```python
from build123d import *

# Parameters (mm, degrees)
F0_W          = 7
F0_H          = 100
F1_DEPTH      = 75
F1_DEPTH_BACK = 75
F2_W          = 7
F2_H          = 125
F3_DEPTH      = 5
F5_R          = 25
F6_R          = 3


with BuildPart() as f1:
    # F0 (on Right) → F1 (new body, two sides)
    with BuildSketch(Plane.YZ) as f1_sk:
        Rectangle(F0_W, F0_H)
    extrude(amount=F1_DEPTH)
    extrude(f1_sk.sketch, amount=-F1_DEPTH_BACK)

    # F2 (on face) → F3 (join)
    with BuildSketch(Plane.YZ.offset(75)):
        with Locations((0, -12.5)):
            Rectangle(F2_W, F2_H)
    extrude(amount=F3_DEPTH)

    # F4: F1 across plane


with BuildPart() as f1_1:
    add(f1.part)
    add(f1.part.mirror(Plane.YZ))

    # F5
    f5_edges = [f1_1.edges().sort_by_distance(p)[0] for p in [
        (-80, 0, 50),
        (80, 0, 50),
    ]]
    fillet(f5_edges, radius=F5_R)

    # F6
    f6_edges = [f1_1.edges().sort_by_distance(p)[0] for p in [
        (-77.5, -3.5, -75),
        (77.5, -3.5, -75),
        (-77.5, 3.5, -75),
        (77.5, 3.5, -75),
    ]]
    fillet(f6_edges, radius=F6_R)


solid = f1_1.part
```
Geometry check sheet. Reference: the model listing, model coordinates, mm. A direction names the side the tool comes from. Round coordinates to 2 decimals unless told otherwise and drop trailing zeros. Loops run counter-clockwise (first coordinate to the right, second up) from the corner with the lowest first, then second, coordinate; pieces in that order, holes last. Notation, with made-up numbers: (61, 54) -> (81, 54) arc R19 cw to (81, 79) -> close; hole circle Ø6 at (61.5, -17). An arc over 180 degrees is marked (long way). Use a Markdown table: item, result.
(1) Sectioned sample at D-D (z = 42.5). Enter the section's corners in (x, y), then the cut area to 3 significant figures.
Calculated:
| item | result |
|---|---|
| outline | (-72.85, -3.5) -> (72.85, -3.5) -> (72.85, 3.5) -> (-72.85, 3.5) -> close |
| area | 1,020 mm² |
(2) Mould release check, pull along X, two halves, no side actions. Record for faces 3 (the flat face through (1, 3.5, 2)), 4 (the flat face through (80, 0, -24)), 5 (the flat face through (-75, 0, -62)), 6 (the flat face through (75, 0, -62)): released by +X, released by -X, zero draft, split by the parting line, or undercut.
Calculated:
| item | result |
|---|---|
| face 3 | zero draft |
| face 4 | released by +X |
| face 5 | undercut |
| face 6 | undercut |
(3) Set-up check for faces 1 (the cylindrical face through (72.871, 0.049, 42.482)), 2 (the flat face through (1, 0, -50)): record each of +Z, -Z, +X, -X, +Y, -Y from which the full face is reachable in a straight line by a thin tool's end or side.
Calculated:
| item | result |
|---|---|
| face 1 | +Z, +X, +Y, -Y |
| face 2 | -Z, +Y, -Y |
(4) Scan lines: probe 1 along X at (y, z) = (0, -53.5); probe 2 along Z at (x, y) = (-43, 3); probe 3 along Z at (x, y) = (-63.5, 2). Record each from-to range of solid material in increasing order.
Calculated:
| item | result |
|---|---|
| probe 1 | -80 to -75, 75 to 80 |
| probe 2 | -50 to 50 |
| probe 3 | -50 to 48.51 |
(5) Go/stop test with a flat-tipped pin: P1, Ø3.5, axis at x = -33.5, y = -0.5, coming from the -Z side. Record where the tip stops, or that it passes through.
Calculated:
| item | result |
|---|---|
| P1 | z = -50 |
(6) Sectioned sample at C-C (y = 2). Enter the section's corners in (x, z).
Calculated:
| item | result |
|---|---|
| outline | (-80, -74.6) -> (-75, -74.6) -> (-75, -50) -> (75, -50) -> (75, -74.6) -> (80, -74.6) -> (80, 25) arc R25 ccw to (55, 50) -> (-55, 50) arc R25 ccw to (-80, 25) -> close |
(7) Sectioned sample at A-A (z = -59.5). Enter the section's corners in (x, y).
Calculated:
| item | result |
|---|---|
| outline | (-80, -3.5) -> (-75, -3.5) -> (-75, 3.5) -> (-80, 3.5) -> close; (75, -3.5) -> (80, -3.5) -> (80, 3.5) -> (75, 3.5) -> close |
(8) Sectioned sample at B-B (x = -18.5). Enter the section's corners in (y, z), then the cut area to 3 significant figures.
Calculated:
| item | result |
|---|---|
| outline | (-3.5, -50) -> (3.5, -50) -> (3.5, 50) -> (-3.5, 50) -> close |
| area | 700 mm² |
